from build123d import *

# Parameters (mm, degrees)
CYLINDER003_R     = 20
CYLINDER003_DEPTH = 10
CYLINDER002_R     = 80
CYLINDER002_DEPTH = 10
BOX006_W          = 300
BOX006_H          = 190
BOX006_DEPTH      = 340


with BuildPart() as cylinder003:
    # Cylinder003 → Cylinder003 (new body)
    with BuildSketch(Plane(origin=(296, 95, 1133), x_dir=(0, 0, -1), z_dir=(1, 0, 0))):
        Circle(CYLINDER003_R)
    extrude(amount=CYLINDER003_DEPTH)


with BuildPart() as cylinder002:
    # Cylinder002 → Cylinder002 (new body)
    with BuildSketch(Plane(origin=(296, 95, 950), x_dir=(0, 0, -1), z_dir=(1, 0, 0))):
        Circle(CYLINDER002_R)
    extrude(amount=CYLINDER002_DEPTH)


with BuildPart() as speaker002:
    # Box006 → Box006 (new body)
    with BuildSketch(Plane.XY.offset(850)):
        with Locations((150, 95)):
            Rectangle(BOX006_W, BOX006_H)
    extrude(amount=BOX006_DEPTH)

    # Cut003: cut Cylinder002
    add(cylinder002.part, mode=Mode.SUBTRACT)

    # Cut002: cut Cylinder003
    add(cylinder003.part, mode=Mode.SUBTRACT)


with BuildPart() as speaker002_1:
    # Cut002 placement: moved
    add(speaker002.part.moved(Location((30, 85, -154))))


solid = speaker002_1.part
Verification items for the finished model (mm, model axes). A direction names the side the tool comes from. Coordinates: 2 decimals unless noted, no trailing zeros. Put each result on its own line as item: value. Start each with the question number.
1. Material ranges on L1, parallel to Z at x = 328, y = 180; L2, parallel to Y at x = 327.95, z = 796; L3, parallel to Y at x = 327.4, z = 979, recorded low to high. Write a range as [from, to].
2. Mould release check, pull along Z, two halves, no side actions. Record for faces 3 (the flat face through (178, 181, 696)), 4 (the cylindrical face through (327.972, 183.517, 875.923)), 5 (the flat face through (178, 275, 864)): released by +Z, released by -Z, zero draft, split by the parting line, or undercut.
3. Access from +Z, -Z, +X, -X, +Y, -Y to the whole of each face (thin tool, end or side, straight path). Record for faces 1 (the flat face through (178, 181, 1036)), 2 (the flat face through (326, 180, 979)).
4. Go/stop test with a flat-tipped pin: pin 1 Ø8 at (y, z) = (148.5, 736) entering from +X. Record where the tip stops, or that it passes through.
Computed:
1. L1: [696, 716], [876, 959], [999, 1036]
1. L2: [85, 100], [260, 275]
1. L3: [85, 160], [200, 275]
2. face 3: released by -Z
2. face 4: undercut
2. face 5: zero draft
3. face 1: +Z, +X, -X, +Y, -Y
3. face 2: +X
4. pin 1: x = 326
